The model under review builds one solid part; all positions refer to its coordinate system, in mm. Coordinates: 2 decimals unless noted, no trailing zeros. Write each loop counter-clockwise with the first axis right and the second up, starting at its lowest first coordinate (ties: lowest second). Pieces come first, ordered by that corner, then holes. Notation, with made-up numbers: (57.25, 14) - (81.25, 14) arc R22 cw to (81.25, 35) - close; hole circle Ø4 at (-21, 7.25). An arc over 180 degrees is marked (long way). Return JSON: item names as keys, results as strings. Group by question number.
(1) We need section B-B on z = 0. State the section outline as (x, y) points, then the cut area to 3 significant figures.
(2) To check wall thickness, follow L1, parallel to X at y = 1.25, z = 0; L2, parallel to X at y = 1.4, z = 2.5; L3, parallel to Z at x = 14, y = 0.9. State the ranges of each line that lie inside material, in increasing order. Write a range as from..to.
(3) We need section D-D on x = -4.5. State the section outline as (y, z) points, then the cut area to 3 significant figures.
(4) For pin 1 Ø0.8 at (x, y) = (-15, 4) entering from -Z; pin 2 Ø2.5 at (x, z) = (25, 0) entering from +Y, all flat-tipped, find the tip position at first contact; note any pin that passes through.
(5) We need section C-C on y = 2.4. State the section outline as (x, z) points.
(6) We need section A-A on x = -25. State the section outline as (y, z) points, then the cut area to 3 significant figures.
```python
from build123d import *

# Parameters (mm, degrees)
SKETCH1_W           = 60
SKETCH1_H           = 40
MAINBODY_DEPTH      = 3
CUT_EXTRUDE1_REACH  = 38.18
SKETCH2_W           = 28.6
SKETCH2_H           = 28
CUT_EXTRUDE2_REACH  = 38.18
SKETCH7_R           = 1.5
SKETCH8_W           = 3
SKETCH8_H           = 3
BOSS_EXTRUDE2_DEPTH = 3
CUT_EXTRUDE3_REACH  = 38.18
SKETCH9_W           = 4.85
SKETCH9_H           = 10
SKETCH9_W_2         = 2
SKETCH10_W          = 2.1
SKETCH10_H          = 6.2
BOSS_EXTRUDE3_DEPTH = 1.5


with BuildPart() as part:
    # Sketch1 → MainBody (new body)
    with BuildSketch(Plane(origin=(0, 0, 0), x_dir=(1, 0, 0), z_dir=(0, 1, 0))):
        Rectangle(SKETCH1_W, SKETCH1_H)
    extrude(amount=MAINBODY_DEPTH)

    # Sketch2 → Cut-Extrude1 (cut, up to next)
    with BuildSketch(Plane(origin=(0, 3, 0), x_dir=(1, 0, 0), z_dir=(0, 1, 0)), mode=Mode.PRIVATE) as cut_extrude1_sk1:
        with Locations((5, 0)):
            Rectangle(SKETCH2_W, SKETCH2_H)
    cut_extrude1_tool1 = extrude(cut_extrude1_sk1.sketch, amount=-CUT_EXTRUDE1_REACH, mode=Mode.PRIVATE) & part.part
    add(cut_extrude1_tool1.solids().sort_by_distance((5, 3, 0))[0], mode=Mode.SUBTRACT)

    # Sketch7 → Cut-Extrude2 (cut, up to next)
    with BuildSketch(Plane(origin=(0, 3, 0), x_dir=(1, 0, 0), z_dir=(0, 1, 0)), mode=Mode.PRIVATE) as cut_extrude2_sk1:
        with Locations(Location((25, 0, 0), (0, 0, 270))):
            Circle(SKETCH7_R)
    cut_extrude2_tool1 = extrude(cut_extrude2_sk1.sketch, amount=-CUT_EXTRUDE2_REACH, mode=Mode.PRIVATE) & part.part
    # Sketch7 → Cut-Extrude2 (cut, up to next)
    with BuildSketch(Plane(origin=(0, 3, 0), x_dir=(1, 0, 0), z_dir=(0, 1, 0)), mode=Mode.PRIVATE) as cut_extrude2_sk2:
        with Locations(Location((-25, 0, 0), (0, 0, 270))):
            Circle(SKETCH7_R)
    cut_extrude2_tool2 = extrude(cut_extrude2_sk2.sketch, amount=-CUT_EXTRUDE2_REACH, mode=Mode.PRIVATE) & part.part
    add(cut_extrude2_tool1.solids().sort_by_distance((25, 3, 0))[0], mode=Mode.SUBTRACT)
    add(cut_extrude2_tool2.solids().sort_by_distance((-25, 3, 0))[0], mode=Mode.SUBTRACT)

    # Sketch8 → Boss-Extrude2 (add)
    with BuildSketch(Plane(origin=(0, 3, 0), x_dir=(1, 0, 0), z_dir=(0, 1, 0))):
        with Locations((-7.8, 12.5)):
            Rectangle(SKETCH8_W, SKETCH8_H)
        with Locations((-7.8, -12.5)):
            Rectangle(SKETCH8_W, SKETCH8_H)
        with Locations((17.8, -12.5)):
            Rectangle(SKETCH8_W, SKETCH8_H)
        with Locations((17.8, 12.5)):
            Rectangle(SKETCH8_W, SKETCH8_H)
    extrude(amount=-BOSS_EXTRUDE2_DEPTH)

    # Sketch9 → Cut-Extrude3 (cut, up to next)
    with BuildSketch(Plane(origin=(0, 3, 0), x_dir=(1, 0, 0), z_dir=(0, 1, 0)), mode=Mode.PRIVATE) as cut_extrude3_sk1:
        with Locations((-11.725, 0)):
            Rectangle(SKETCH9_W, SKETCH9_H)
    cut_extrude3_tool1 = extrude(cut_extrude3_sk1.sketch, amount=-CUT_EXTRUDE3_REACH, mode=Mode.PRIVATE) & part.part
    # Sketch9 → Cut-Extrude3 (cut, up to next)
    with BuildSketch(Plane(origin=(0, 3, 0), x_dir=(1, 0, 0), z_dir=(0, 1, 0)), mode=Mode.PRIVATE) as cut_extrude3_sk2:
        with Locations((-17.25, 0)):
            Rectangle(SKETCH9_W_2, SKETCH9_H)
    cut_extrude3_tool2 = extrude(cut_extrude3_sk2.sketch, amount=-CUT_EXTRUDE3_REACH, mode=Mode.PRIVATE) & part.part
    add(cut_extrude3_tool1.solids().sort_by_distance((-11.725, 3, 0))[0], mode=Mode.SUBTRACT)
    add(cut_extrude3_tool2.solids().sort_by_distance((-17.25, 3, 0))[0], mode=Mode.SUBTRACT)

    # Sketch10 → Boss-Extrude3 (add)
    with BuildSketch(Plane(origin=(0, 3, 0), x_dir=(1, 0, 0), z_dir=(0, 1, 0))):
        with Locations((-15.2, 0)):
            Rectangle(SKETCH10_W, SKETCH10_H)
    extrude(amount=BOSS_EXTRUDE3_DEPTH)


solid = part.part
```
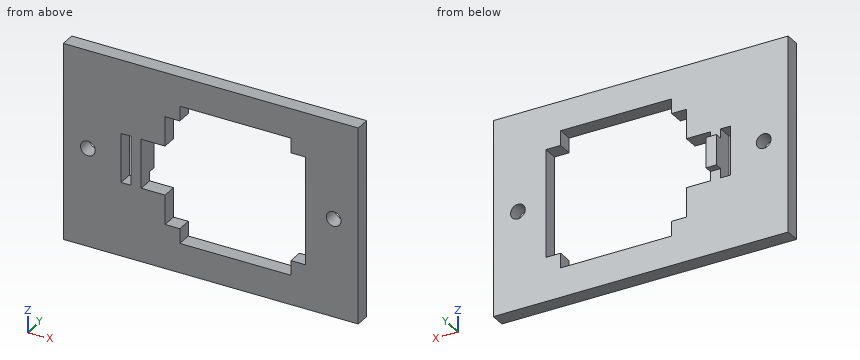
Ans:
{
 "1": {"outline": "(-30, 0) - (-26.5, 0) - (-26.5, 3) - (-30, 3) - close; (-23.5, 0) - (-18.25, 0) - (-18.25, 3) - (-23.5, 3) - close; (-16.25, 0) - (-14.15, 0) - (-14.15, 4.5) - (-16.25, 4.5) - close; (19.3, 0) - (23.5, 0) - (23.5, 3) - (19.3, 3) - close; (26.5, 0) - (30, 0) - (30, 3) - (26.5, 3) - close", "area": "58.8 mm²"},
 "2": {"L1": "-30..-26.5, -23.5..-18.25, -16.25..-14.15, 19.3..23.5, 26.5..30", "L2": "-30..-18.25, -16.25..-14.15, 19.3..30", "L3": "-20..-14, 14..20"},
 "3": {"outline": "(0, -20) - (3, -20) - (3, -14) - (0, -14) - close; (0, 14) - (3, 14) - (3, 20) - (0, 20) - close", "area": "36.0 mm²"},
 "4": {"pin 1": "z = -3.1", "pin 2": "through"},
 "5": {"outline": "(-30, -20) - (30, -20) - (30, 20) - (-30, 20) - close; hole circle Ø3 at (-25, 0); hole (-18.25, -5) - (-16.25, -5) - (-16.25, 5) - (-18.25, 5) - close; hole (-14.15, -5) - (-9.3, -5) - (-9.3, -11) - (-6.3, -11) - (-6.3, -14) - (16.3, -14) - (16.3, -11) - (19.3, -11) - (19.3, 11) - (16.3, 11) - (16.3, 14) - (-6.3, 14) - (-6.3, 11) - (-9.3, 11) - (-9.3, 5) - (-14.15, 5) - close; hole circle Ø3 at (25, 0)"},
 "6": {"outline": "(0, -20) - (3, -20) - (3, -1.5) - (0, -1.5) - close; (0, 1.5) - (3, 1.5) - (3, 20) - (0, 20) - close", "area": "111 mm²"}
}
